The model under review builds one solid part; all positions refer to its coordinate system, in mm. Face numbers are marked on the shaded views. Coordinates: 2 decimals unless noted, no trailing zeros. Order: outer loops, then holes, each group sorted by start corner. A loop starts at its lowest first (then second) coordinate and runs counter-clockwise, first axis right, second up. Notation, with made-up numbers: M 3.5,25 L 8.5,25 A27 ccw 8.5,48 Z; hole C 38,64 d5. An arc over 180 degrees is marked long. One line per item, written item: value.
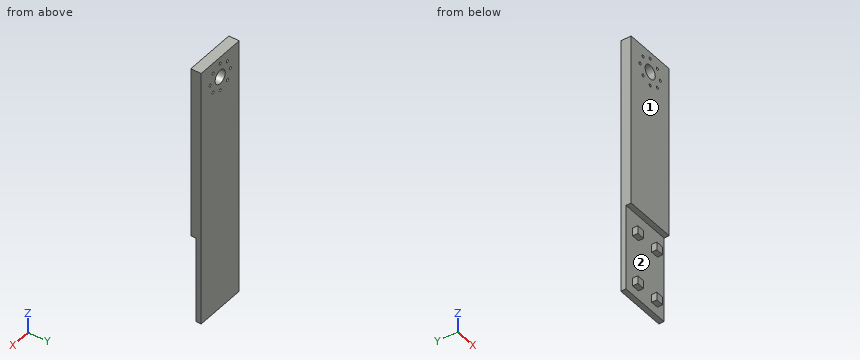
```python
from build123d import *

# Parameters (mm, degrees)
F0_W     = 30
F0_H     = 6
F1_DEPTH = 150
F2_R     = 0.8
F2_R_2   = 4
F3_DEPTH = 6
F4_W     = 3
F4_H     = 50
F5_DEPTH = 30
F6_W     = 4.604
F6_H     = 4.608
F6_W_2   = 4.599998
F6_H_2   = 4.599998
F6_W_3   = 4.591
F6_H_3   = 4.59
F6_W_4   = 4.592
F6_H_4   = 4.592
F7_DEPTH = 3


with BuildPart() as f1:
    # F0 (on Top) → F1 (new body)
    with BuildSketch(Plane.XY):
        Rectangle(F0_W, F0_H)
    extrude(amount=F1_DEPTH)

    # F2 (on face) → F3 (cut, through all)
    with BuildSketch(Plane.XZ.offset(3)):
        with Locations((0, 146.2)):
            Circle(F2_R)
        with Locations((0, 138.2)):
            Circle(F2_R_2)
        with Locations((-5.656854, 143.856854)):
            Circle(F2_R)
        with Locations((-8, 138.2)):
            Circle(F2_R)
        with Locations((-5.656854, 132.543146)):
            Circle(F2_R)
        with Locations((0, 130.2)):
            Circle(F2_R)
        with Locations((5.656854, 132.543146)):
            Circle(F2_R)
        with Locations((8, 138.2)):
            Circle(F2_R)
        with Locations((5.656854, 143.856854)):
            Circle(F2_R)
    extrude(amount=-F3_DEPTH, mode=Mode.SUBTRACT)

    # F4 (on face) → F5 (cut, through all)
    with BuildSketch(Plane(origin=(-15, 0, 0), x_dir=(0, -1, 0), z_dir=(-1, 0, 0))):
        with Locations((1.5, 25)):
            Rectangle(F4_W, F4_H)
    extrude(amount=-F5_DEPTH, mode=Mode.SUBTRACT)

    # F6 (on face) → F7 (join)
    with BuildSketch(Plane.XZ):
        with Locations((-7.502, 37.5)):
            Rectangle(F6_W, F6_H)
        with Locations((7.5, 37.5)):
            Rectangle(F6_W_2, F6_H_2)
        with Locations((-7.4995, 7.5)):
            Rectangle(F6_W_3, F6_H_3)
        with Locations((7.5, 7.5)):
            Rectangle(F6_W_4, F6_H_4)
    extrude(amount=F7_DEPTH)


solid = f1.part
```
(1) Mouldability with a two-part tool opening along Z and no side actions: class the marked faces 1 and 2 as +Z half, -Z half, draft (parallel to the pull), parting line (faces both ways), or undercut.
Geometry results:
face 1: draft
face 2: undercut
(2) We need section C-C, the plane z = 47.5. State the section outline as (x, y) points.
Geometry results:
outline: M -15,0 L 15,0 L 15,3 L -15,3 Z
(3) We need section A-A, the plane y = -0.9. Count the separate pieces of the cut face and the enclosed holes in it, plus the area to 3 significant figures.
Geometry results:
separate pieces: 5
enclosed holes: 9
area: 3,020 mm2
(4) For L1, parallel to Z at x = 0, y = 0.55; L2, parallel to Z at x = -8, y = -0.6 (3 decimals); L3, parallel to Z at x = 8, y = 1.2, list the stretches that pass through material, from the lowest coordinate up.
Geometry results:
L1: z = 0 to 129.4, 131 to 134.2, 142.2 to 145.4, 147 to 150
L2: z = 5.205 to 9.795, 35.196 to 39.804, 50 to 137.4, 139 to 150
L3: z = 0 to 137.4, 139 to 150
(5) We need section B-B, the plane x = 11.75. State the section outline as (y, z) points, plus the area to 3 significant figures.
Geometry results:
outline: M -3,50 L 0,50 L 0,0 L 3,0 L 3,150 L -3,150 Z
area: 750 mm2
(6) Insertion check: pin 1 Ø0.9 at (y, z) = (-1.5, 38) entering from +X; pin 2 Ø1.5 at (y, z) = (-1.5, 37) entering from -X; pin 3 Ø1.5 at (x, y) = (7, -1) entering from -Z. Each pin has a flat end and moves straight along its axis. Give the tip position at first contact, or say it passes through.
Geometry results:
pin 1: stops at x = 9.8
pin 2: stops at x = -9.8
pin 3: stops at z = 5.2
